Part model, mm, in its own coordinate system. Face numbers are marked on the shaded views. Round coordinates to 2 decimals unless told otherwise and drop trailing zeros. Loops run counter-clockwise (first coordinate to the right, second up) from the corner with the lowest first, then second, coordinate; pieces in that order, holes last. Notation, with made-up numbers: (72.25, 33) -> (104.25, 33) arc R8 ccw to (104.25, 48) -> close; hole circle Ø10 at (73.5, 63.25). An arc over 180 degrees is marked (long way). Use a Markdown table: item, result. Add a question column.
Item 1: Probe line 1 (Y direction, x = 0, z = 0); line 2 (X direction, y = 1, z = 3.5); line 3 (Y direction, x = 2.7, z = 1). List the from-to ranges inside material, lowest first. Write a range as [from, to].
Item 2: Cut at C-C, the plane z = 0.25. List the corners of the cut face in (x, y), plus the area to 3 significant figures.
Item 3: Cut at B-B, the plane x = 0. List the corners of the cut face in (y, z), plus the area to 3 significant figures.
Item 4: Cut at A-A, the plane y = 0. List the corners of the cut face in (x, z).
Item 5: Cut at D-D, the plane z = 3. List the corners of the cut face in (x, y), plus the area to 3 significant figures.
Item 6: Two-plate mould, pull along Y, no slides. Class the marked faces 1, 2, 3 and 4: pulls with the +Y half, pulls with the -Y half, needs draft (parallel to the pull), parting line crosses it, or undercut.
Item 7: Flat gauge pins, fed straight in: pin 1 (1.5 mm diameter, centred on y = -8.5, z = 0, fed in from -X); pin 2 (3 mm diameter, centred on y = 8.5, z = 0, fed in from +X). Where does each tip first touch, or does it go through?
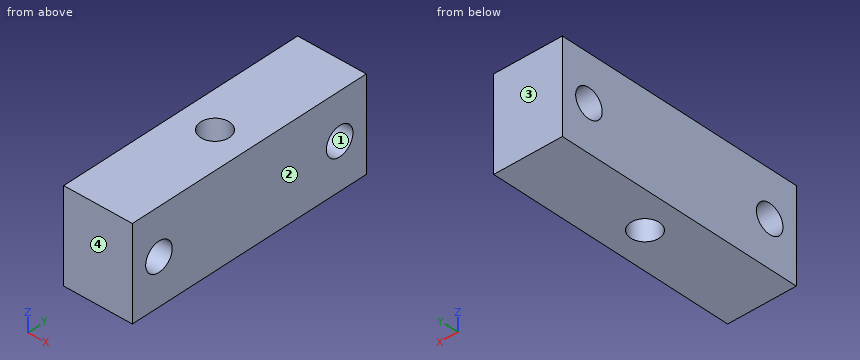
```python
from build123d import *

# Parameters (mm, degrees)
SKETCH_1_W          = 6
SKETCH_1_H          = 8
EXTRUDE_1_DEPTH     = 11
SKETCH_2_R          = 1.25
CUT_EXTRUDE_1_DEPTH = 14.928388277
SKETCH_3_R          = 1.25
CUT_EXTRUDE_2_DEPTH = 14.152946438


with BuildPart() as part:
    # 草图1 → 凸台-拉伸1 (new, symmetric)
    with BuildSketch(Plane(origin=(0, 0, 0), x_dir=(1, 0, 0), z_dir=(0, 1, 0))):
        Rectangle(SKETCH_1_W, SKETCH_1_H)
    extrude(amount=EXTRUDE_1_DEPTH, both=True)

    # 草图2 → 切除-拉伸1 (cut, through all)
    with BuildSketch(Plane.XY.offset(4)):
        Circle(SKETCH_2_R)
    extrude(amount=-CUT_EXTRUDE_1_DEPTH, mode=Mode.SUBTRACT)

    # 草图3 → 切除-拉伸2 (cut, through all)
    with BuildSketch(Plane.ZY.offset(3)):
        with Locations((0, 8.5)):
            Circle(SKETCH_3_R)
        with Locations((0, -8.5)):
            Circle(SKETCH_3_R)
    extrude(amount=-CUT_EXTRUDE_2_DEPTH, mode=Mode.SUBTRACT)


solid = part.part
```
A:
| question | item | result |
|---|---|---|
| 1 | line 1 | y = [-11, -9.75], [-7.25, -1.25], [1.25, 7.25], [9.75, 11] |
| 1 | line 2 | x = [-3, -0.75], [0.75, 3] |
| 1 | line 3 | y = [-11, -9.25], [-7.75, 7.75], [9.25, 11] |
| 2 | outline | (-3, -11) -> (3, -11) -> (3, -9.72) -> (-3, -9.72) -> close; (-3, -7.28) -> (3, -7.28) -> (3, 7.28) -> (-3, 7.28) -> close; (-3, 9.72) -> (3, 9.72) -> (3, 11) -> (-3, 11) -> close; hole circle Ø2.5 at (0, 0) |
| 2 | area | 97.7 mm^2 |
| 3 | outline | (-11, -4) -> (-1.25, -4) -> (-1.25, 4) -> (-11, 4) -> close; (1.25, -4) -> (11, -4) -> (11, 4) -> (1.25, 4) -> close; hole circle Ø2.5 at (-8.5, 0); hole circle Ø2.5 at (8.5, 0) |
| 3 | area | 146 mm^2 |
| 4 | outline | (-3, -4) -> (-1.25, -4) -> (-1.25, 4) -> (-3, 4) -> close; (1.25, -4) -> (3, -4) -> (3, 4) -> (1.25, 4) -> close |
| 5 | outline | (-3, -11) -> (3, -11) -> (3, 11) -> (-3, 11) -> close; hole circle Ø2.5 at (0, 0) |
| 5 | area | 127 mm^2 |
| 6 | face 1 | undercut |
| 6 | face 2 | needs draft |
| 6 | face 3 | pulls with the +Y half |
| 6 | face 4 | pulls with the -Y half |
| 7 | pin 1 | passes through |
| 7 | pin 2 | stops at x = 3 |
